Model file for the job. Use its own axes, mm. A direction names the side the tool comes from. Give positions to 0.01 mm unless a question says otherwise; leave off trailing zeros. Write each loop counter-clockwise with the first axis right and the second up, starting at its lowest first coordinate (ties: lowest second). Pieces come first, ordered by that corner, then holes. Notation, with made-up numbers: (8, -24.5) - (34, -24.5) arc R14 ccw to (34, 0.5) - close; hole circle Ø10 at (45.5, -0.75). An arc over 180 degrees is marked (long way). One line per item, written item: value. Start each with the question number.
(1) Mould opens along Y. For faces 1 (the face through (3.5, 0.1, 110.8)), 2 (the face through (3.46, -114.19, 5.03)), 3 (the face through (22.436, 20, 40)) say: pulls with the +Y half, pulls with the -Y half, needs draft (parallel to the pull), parting line crosses it, or undercut.
(2) Cut at A-A, the plane z = 108.2. List the corners of the cut face in (x, y).
(3) Probe L1, parallel to Z at x = 1.5, y = -89; L2, parallel to X at y = -82.5, z = -66; L3, parallel to Z at x = 10.5, y = 0. List the from-to ranges inside material, lowest first.
(4) Drop flat-ended pins along their axis: P1, Ø7, axis at y = 0, z = -108.2, coming from the +X side; P2, Ø4, axis at x = 7, y = -26, coming from the +Z side; P3, Ø8.5, axis at y = 108.2, z = 0, coming from the -X side. Give the stop position or say it passes through.
(5) 3-axis set-ups, long thin cutter, end or side, ignore diameter. For faces 4 (the face through (1.76, -82.531, -63.282)), 5 (the face through (3.46, -95.29, -52.04)), 6 (the face through (17.045, -34.908, -26.767)): which of +Z, -Z, +X, -X, +Y, -Y reach the whole face in a straight line?
(6) Cut at C-C, the plane z = 0. State how many separate pieces and enclosed holes the cut face has, and give its area (3 significant figures).
from build123d import *

# Parameters (mm, degrees)
SKETCH2_R          = 2.6
CUT_EXTRUDE1_DEPTH = 10


with BuildPart() as part:
    # Sketch1 → Revolve1 (revolve)
    with BuildSketch(Plane.XY):
        Polygon((0, 27.5), (10, 27.5), (10, 27), (11.5, 27), (11.5, 43.989032899), (22.436374316, 43.989032899), (22.436374316, 53.08402355), (6, 53.08402355), (6, 114.3), (1, 114.3), (1, 104), (2.5, 104), (2.5, 102.5), (0.5, 102.5), (-0.5, 102.2), (-0.5, 100.5), (2.5, 100.5), (5, 98.23), (5, 73.23), (0, 35.229488808), align=None)
    revolve(axis=Axis((0, 0, 0), (1, 0, 0)))

    # Sketch2 → Cut-Extrude1 (cut)
    with BuildSketch(Plane(origin=(0, 0, 0), x_dir=(0, 0, -1), z_dir=(1, 0, 0))):
        with Locations((0, 108.2)):
            Circle(SKETCH2_R)
        with Locations((54.1, 93.703948689)):
            Circle(SKETCH2_R)
        with Locations((93.703948689, 54.1)):
            Circle(SKETCH2_R)
        with Locations((108.2, 0)):
            Circle(SKETCH2_R)
        with Locations((93.703948689, -54.1)):
            Circle(SKETCH2_R)
        with Locations((54.1, -93.703948689)):
            Circle(SKETCH2_R)
        with Locations((0, -108.2)):
            Circle(SKETCH2_R)
        with Locations((-54.1, -93.703948689)):
            Circle(SKETCH2_R)
        with Locations((-93.703948689, -54.1)):
            Circle(SKETCH2_R)
        with Locations((-108.2, 0)):
            Circle(SKETCH2_R)
        with Locations((-93.703948689, 54.1)):
            Circle(SKETCH2_R)
        with Locations((-54.1, 93.703948689)):
            Circle(SKETCH2_R)
    extrude(amount=CUT_EXTRUDE1_DEPTH, mode=Mode.SUBTRACT)


solid = part.part
Answers follow:
1. face 1: undercut
1. face 2: parting line crosses it
1. face 3: needs draft
2. outline: (1, -36.84) - (6, -36.84) - (6, -2.6) - (1, -2.6) - close; (1, 2.6) - (6, 2.6) - (6, 36.84) - (1, 36.84) - close
3. L1: z = -71.72 to -53.81, -50.85 to -46.68, 46.68 to 50.85, 53.81 to 71.72
3. L2: x = 1 to 6
3. L3: z = -53.08 to -27, 27 to 53.08
4. P1: stops at x = 6
4. P2: stops at z = 111.69
4. P3: stops at x = 1
5. face 4: -X
5. face 5: +X, -X
5. face 6: +X
6. separate pieces: 4
6. enclosed holes: 0
6. area: 988 mm²
